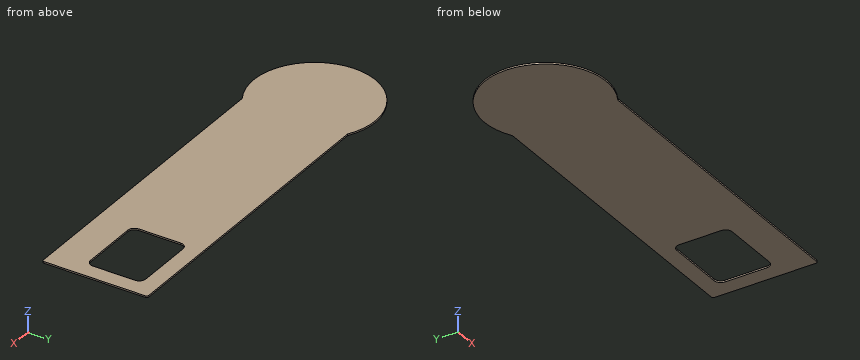
from build123d import *

# Parameters (mm, degrees)
F0_W     = 551.17
F0_H     = 155.58
F1_DEPTH = 2.38125
F2_R     = 3
F3_W     = 105
F3_H     = 81.79
F4_DEPTH = 25
F5_R     = 10
F6_R     = 90
F7_DEPTH = 2.38125


# Not quite as in the source:
# - a length typed as a fraction of an inch, garbled in the dataset ("3 / 203.2 mm" for 3/8 in), is restored


with BuildPart() as f1:
    # F0 (on Top) → F1 (new body)
    with BuildSketch(Plane.XY):
        Rectangle(F0_W, F0_H)
    extrude(amount=F1_DEPTH)

    # F2
    f2_edges = [f1.edges().sort_by_distance(p)[0] for p in [
        (275.585, -77.79, 1.190625),
        (-275.585, -77.79, 1.190625),
        (-275.585, 77.79, 1.190625),
        (275.585, 77.79, 1.190625),
    ]]
    fillet(f2_edges, radius=F2_R)

    # F3 (on face) → F4 (cut)
    with BuildSketch(Plane.XY.offset(2.38125)):
        with Locations((199.085, 12.895)):
            Rectangle(F3_W, F3_H)
    extrude(amount=-F4_DEPTH, mode=Mode.SUBTRACT)

    # F5
    f5_edges = [f1.edges().sort_by_distance(p)[0] for p in [
        (146.585, 53.79, 1.190625),
        (146.585, -28, 1.190625),
        (251.585, 53.79, 1.190625),
        (251.585, -28, 1.190625),
    ]]
    fillet(f5_edges, radius=F5_R)

    # F6 (on face) → F7 (join, through all)
    with BuildSketch(Plane.XY.offset(2.38125)):
        with Locations((-228.1388989337, 0)):
            Circle(F6_R)
    extrude(amount=-F7_DEPTH)


solid = f1.part
The model under review builds one solid part; all positions refer to its coordinate system, in mm. Round coordinates to 2 decimals unless told otherwise and drop trailing zeros. Order: outer loops, then holes, each group sorted by start corner. A loop starts at its lowest first (then second) coordinate and runs counter-clockwise, first axis right, second up. Notation, with made-up numbers: (7, -35) -> (23, -35) arc R17 ccw to (23, -20) -> close; hole circle Ø2 at (1, -22). An arc over 180 degrees is marked (long way). Return JSON: item names as keys, results as strings.
1. Insertion check: P1, Ø0.7, axis at x = 208.5, z = 1, coming from the -Y side; P2, Ø1, axis at x = -142, z = 2, coming from the +Y side; P3, Ø1.2, axis at y = 21.5, z = 1, coming from the -X side. Each pin has a flat end and moves straight along its axis. Give the tip position at first contact, or say it passes through.
Answer block:
{"P1": "stops at y = -77.79", "P2": "stops at y = 77.79", "P3": "stops at x = -315.68"}
2. Take a section at D-D (x = -134). Write out the cut boundary in (y, z).
Answer block:
{"outline": "(-77.79, 0) -> (77.79, 0) -> (77.79, 2.38) -> (-77.79, 2.38) -> close"}
3. Take a section at C-C (z = 0.8). Write out the cut boundary in (x, y) (3 decimals), then the cut area to 3 significant figures.
Answer block:
{"outline": "(-182.876, -77.79) -> (272.585, -77.79) arc R3 ccw to (275.585, -74.79) -> (275.585, 74.79) arc R3 ccw to (272.585, 77.79) -> (-182.876, 77.79) arc R90 ccw (long way) to start; hole (146.585, -18) arc R10 ccw to (156.585, -28) -> (241.585, -28) arc R10 ccw to (251.585, -18) -> (251.585, 43.79) arc R10 ccw to (241.585, 53.79) -> (156.585, 53.79) arc R10 ccw to (146.585, 43.79) -> close", "area": "83,300 mm²"}
4. Take a section at B-B (x = 235). Write out the cut boundary in (y, z).
Answer block:
{"outline": "(-77.79, 0) -> (-28, 0) -> (-28, 2.38) -> (-77.79, 2.38) -> close; (53.79, 0) -> (77.79, 0) -> (77.79, 2.38) -> (53.79, 2.38) -> close"}
5. For L1, parallel to Y at x = 234.5, z = 0.85; L2, parallel to X at y = 2, z = 1.1 (3 decimals); L3, parallel to Y at x = 82.5, z = 1.55, list the stretches that pass through material, from the lowest coordinate up. Write a range as [from, to].
Answer block:
{"L1": "y = [-77.79, -28], [53.79, 77.79]", "L2": "x = [-318.117, 146.585], [251.585, 275.585]", "L3": "y = [-77.79, 77.79]"}
6. Take a section at A-A (y = 0). Write out the cut boundary in (x, z) (3 decimals).
Answer block:
{"outline": "(-318.139, 0) -> (146.585, 0) -> (146.585, 2.381) -> (-318.139, 2.381) -> close; (251.585, 0) -> (275.585, 0) -> (275.585, 2.381) -> (251.585, 2.381) -> close"}
